Source: CAD feature listing. Evaluate the final solid. Frame: model axes, mm. A direction names the side the tool comes from. Coordinates: 2 decimals unless noted, no trailing zeros. Order: outer loops, then holes, each group sorted by start corner. A loop starts at its lowest first (then second) coordinate and runs counter-clockwise, first axis right, second up.
```python
from build123d import *

# Parameters (mm, degrees)
REVOLVE_ONTO_SKETCH002_ROLL_ANGLE = 90
ARRAY_COUNT                       = 4
PAD_DEPTH                         = 2
POLARPATTERN_COUNT                = 4
SKETCH005_R                       = 1.6
POCKET_DEPTH                      = 5.001
SKETCH007_W                       = 5
SKETCH007_H                       = 3
POCKET001_DEPTH                   = 5.001
SKETCH008_R                       = 2
POCKET002_DEPTH                   = 4
SKETCH009_R                       = 1.75
POCKET003_DEPTH                   = 5.001
SKETCH010_R                       = 2.7
POCKET004_DEPTH                   = 3.5


with BuildPart() as array:
    # Sketch002 as drawn → Revolve (revolve)
    with BuildSketch(Plane.XY):
        Polygon((17.25, -1), (17.25, 4), (18.5, 4), (18.5, 8), (20, 8), (20, -1), align=None)
    revolve(axis=Axis((20, 8, 0), (0, -1, 0)))


with BuildPart() as array_1:
    # Revolve onto Sketch002 roll: moved
    add(array.part.rotate(Axis((0, 0, 0), (1, 0, 0)), REVOLVE_ONTO_SKETCH002_ROLL_ANGLE))


with BuildPart() as array_2:
    # Revolve onto Sketch002 placement: moved
    add(array_1.part)

    # Array: Array ×4 about axis
    array_axis = Axis((0, 0, 0), (0, 0, 1))


with BuildPart() as array_3:
    add(array_2.part)
    for i in range(1, ARRAY_COUNT):
        add(array_2.part.rotate(array_axis, i * 360 / ARRAY_COUNT))


with BuildPart() as pocket004:
    # Sketch → Revolution (revolve)
    with BuildSketch(Plane.XZ):
        Polygon((0, 0), (24, 0), (24, 7), (22, 7), (22, 5), (8.6, 5), (8.6, 7), (6.6, 7), (6.6, 2), (0, 2), align=None)
    revolve(axis=Axis((0, 0, 0), (0, 0, 1)))

    # Sketch004 → Pad (new body)
    with BuildSketch(Plane(origin=(0, 0, 7), x_dir=(-1, 0, 0), z_dir=(0, 0, 1))):
        with BuildLine():
            Line((3, -22), (-3, -22))
            Line((-3, -22), (-3, -20))
            ThreePointArc((3, -20), (0, -17), (-3, -20))
            Line((3, -20), (3, -22))
        make_face()
    pad = extrude(amount=-PAD_DEPTH)

    # PolarPattern: Pad ×4 about axis
    polarpattern_axis = Axis((0, 0, 7), (0, 0, 1))
    for i in range(1, POLARPATTERN_COUNT):
        add(pad.rotate(polarpattern_axis, i * 360 / POLARPATTERN_COUNT))

    # Cut: cut Array
    add(array_3.part, mode=Mode.SUBTRACT)

    # Sketch005 → Pocket (cut, through all)
    with BuildSketch(Plane.XY.offset(5)):
        with Locations((-10, 10)):
            Circle(SKETCH005_R)
        with Locations((10, 10)):
            Circle(SKETCH005_R)
        with Locations((10, -10)):
            Circle(SKETCH005_R)
        with Locations((-10, -10)):
            Circle(SKETCH005_R)
    extrude(amount=-POCKET_DEPTH, mode=Mode.SUBTRACT)

    # Sketch007 → Pocket001 (cut, through all)
    with BuildSketch(Plane.XY.offset(5)):
        with Locations((0, 13.5)):
            Rectangle(SKETCH007_W, SKETCH007_H)
    extrude(amount=-POCKET001_DEPTH, mode=Mode.SUBTRACT)

    # Sketch008 → Pocket002 (cut)
    with BuildSketch(Plane.XY.offset(5)):
        with Locations((-10, 10)):
            Circle(SKETCH008_R)
        with Locations((10, 10)):
            Circle(SKETCH008_R)
        with Locations((10, -10)):
            Circle(SKETCH008_R)
        with Locations((-10, -10)):
            Circle(SKETCH008_R)
    extrude(amount=-POCKET002_DEPTH, mode=Mode.SUBTRACT)

    # Sketch009 → Pocket003 (cut, through all)
    with BuildSketch(Plane.XY.offset(5)):
        with Locations((9.439876, 15.450283)):
            Circle(SKETCH009_R)
        with Locations((15.450283, 9.439876)):
            Circle(SKETCH009_R)
    extrude(amount=-POCKET003_DEPTH, mode=Mode.SUBTRACT)

    # Sketch010 → Pocket004 (cut)
    with BuildSketch(Plane(origin=(0, 0, 0), x_dir=(1, 0, 0), z_dir=(0, 0, -1))):
        with Locations((15.450283, -9.439876)):
            Circle(SKETCH010_R)
        with Locations((9.439876, -15.450283)):
            Circle(SKETCH010_R)
    extrude(amount=-POCKET004_DEPTH, mode=Mode.SUBTRACT)


solid = pocket004.part
```
1. Section query C-C, the plane x = -10. Output: boundary loops of the cut face in (y, z).
2. Material intervals for line 1 along Y through (x, z) = (9.5, 4); line 2 along Y through (x, z) = (10, 3.2); line 3 along Z through (x, y) = (-11, 15), sorted ascending.
3. Access query for faces 4 (the flat face through (14, 8, 3.5)), 5 (the cylindrical face through (10, 12, 3)), 6 (the flat face through (2.5, 13, 3)). Directions: +Z, -Z, +X, -X, +Y, -Y. A direction counts if a zero-diameter tool reaches every point of the face in a straight line with its end or side. Return the directions, or none.
4. Draft query along X for faces 1 (the cylindrical face through (-11.27, -10.97, 0.51)), 2 (the flat face through (2.5, -6.3, 7)), 3 (the cylindrical face through (-23.977, 1.055, 3.549)). Return one class per face: +X half, -X half, draft (parallel to the pull), parting line (faces both ways), or undercut.
5. Section query D-D, the plane y = 4. Output: boundary loops of the cut face in (x, z), plus the area to 3 significant figures.
6. Contact query for flat-ended pins moving along their axis: P1, Ø6, axis at x = 15.45, y = 9.44, coming from the +Z side; P2, Ø4, axis at x = -1, z = 3, coming from the +Y side; P3, Ø1.4, axis at x = 21, z = 6.5, coming from the -Y side. Output: stop coordinate, or through.
7. Section query A-A, the plane x = 10. Count the separate pieces of the cut face and the enclosed holes in it, plus the area to 3 significant figures.
Answer key:
1. outline: (-21.82, 0) - (-11.6, 0) - (-11.6, 1) - (-12, 1) - (-12, 5) - (-19.6, 5) - (-19.6, 7) - (-21.82, 7) - close; (-8.4, 0) - (8.4, 0) - (8.4, 1) - (8, 1) - (8, 5) - (-8, 5) - (-8, 1) - (-8.4, 1) - close; (11.6, 0) - (21.82, 0) - (21.82, 7) - (19.6, 7) - (19.6, 5) - (12, 5) - (12, 1) - (11.6, 1) - close
2. line 1: y = -22.04 to -11.94, -8.06 to 8.06, 11.94 to 13.7, 17.2 to 22.04
2. line 2: y = -21.82 to -12, -8 to 8, 12 to 12.81, 18.09 to 21.82
2. line 3: z = 0 to 5
3. face 4: -Z
3. face 5: +Z
3. face 6: +Z, -Z
4. face 1: undercut
4. face 2: draft
4. face 3: parting line
5. outline: (-23.66, 0) - (23.66, 0) - (23.66, 7) - (21.63, 7) - (21.63, 5) - (7.61, 5) - (7.61, 7) - (5.25, 7) - (5.25, 2) - (-5.25, 2) - (-5.25, 7) - (-7.61, 7) - (-7.61, 5) - (-21.63, 5) - (-21.63, 7) - (-23.66, 7) - close
5. area: 223 mm2
6. P1: stops at z = 5
6. P2: stops at y = 24
6. P3: stops at y = -12.8
7. separate pieces: 4
7. enclosed holes: 0
7. area: 165 mm2
